Read the model definition and answer for the solid it produces. Units are mm, in the model's axes. Give positions to 0.01 mm unless a question says otherwise; leave off trailing zeros. Write each loop counter-clockwise with the first axis right and the second up, starting at its lowest first coordinate (ties: lowest second). Pieces come first, ordered by that corner, then holes. Notation, with made-up numbers: (31.25, 35.5) -> (36.25, 35.5) arc R34 ccw to (36.25, 65.5) -> close; hole circle Ø5 at (36.25, -35.75). An arc over 180 degrees is marked (long way). Use a Markdown table: item, result.
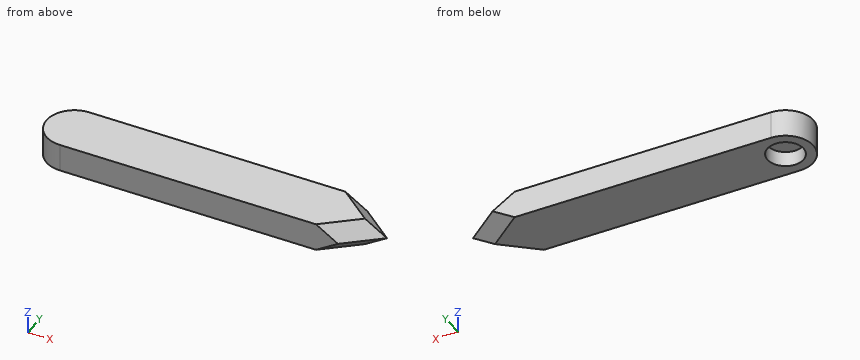
from build123d import *

# Parameters (mm, degrees)
EXTRUDE_1_DEPTH     = 4
SKETCH_2_R          = 2.6
CUT_EXTRUDE_1_DEPTH = 2.2
CHAMFER_2_SIZE      = 2


with BuildPart() as part:
    # 草图1 → 凸台-拉伸1 (new body)
    with BuildSketch(Plane.XY):
        with BuildLine():
            Line((0, 4), (40, 4))
            Line((40, 4), (44.926117642, 0))
            Line((44.926117642, 0), (40, -4))
            Line((40, -4), (0, -4))
            ThreePointArc((0, -4), (-4, 0), (0, 4))
        make_face()
    extrude(amount=EXTRUDE_1_DEPTH)

    # 草图2 → 切除-拉伸1 (cut)
    with BuildSketch(Plane(origin=(0, 0, 0), x_dir=(-1, 0, 0), z_dir=(0, 0, -1))):
        Circle(SKETCH_2_R)
    extrude(amount=-CUT_EXTRUDE_1_DEPTH, mode=Mode.SUBTRACT)

    # 倒角2
    chamfer_2_edges = [part.edges().sort_by_distance(p)[0] for p in [
        (42.463058821, -2, 0),
        (42.463058821, 2, 0),
        (42.463058821, -2, 4),
        (42.463058821, 2, 4),
    ]]
    chamfer(chamfer_2_edges, length=CHAMFER_2_SIZE - 0.0001)  # a hair under: the kernel refuses the full size


solid = part.part
Item 1: Straight lines are drawn through the part: line 1 along Y through (x, z) = (0, 0.85); line 2 along X through (y, z) = (1, 1.9); line 3 along X through (y, z) = (0.5, 0.3). For each, find the intervals that lie inside material, in ascending order. Write a range as [from, to].
Return value:
| item | result |
|---|---|
| line 1 | [-4, -2.6], [2.6, 4] |
| line 2 | [-3.87, -2.4], [2.4, 43.54] |
| line 3 | [-3.97, -2.55], [2.55, 41.61] |
Item 2: A cutting plane is placed at A-A (z = 1.25). Give the vertices of the cut face in (x, y), then the cut area to 3 significant figures.
Return value:
| item | result |
|---|---|
| outline | (0, -4) -> (38.81, -4) -> (43.74, 0) -> (38.81, 4) -> (0, 4) arc R4 ccw to start; hole circle Ø5.2 at (0, 0) |
| area | 334 mm^2 |
Item 3: A cutting plane is placed at C-C (z = 3.3). Give the vertices of the cut face in (x, y).
Return value:
| item | result |
|---|---|
| outline | (0, -4) -> (37.94, -4) -> (42.86, 0) -> (37.94, 4) -> (0, 4) arc R4 ccw to start |
Item 4: This flat-tipped pin is pushed along its axis until it touches: P1, Ø4, axis at x = -0.5, y = 0, coming from the -Z side. Where does it stop, or does it pass through?
Return value:
| item | result |
|---|---|
| P1 | z = 2.2 |
